from build123d import *

# Parameters (mm, degrees)
SKETCH1_W                       = 300
SKETCH1_H                       = 800
BOSS_EXTRUDE1_DEPTH             = 1
SKETCH2_W                       = 3
SKETCH2_H                       = 20
CUT_EXTRUDE1_DEPTH              = 10
EDGE_FLANGE1_STRIP_W            = 6
EDGE_FLANGE1_STRIP_H            = 1
EDGE_FLANGE1_STRIP_CUT_DEPTH    = 3
EDGE_FLANGE1_STRIP_2_W          = 6
EDGE_FLANGE1_STRIP_2_H          = 1
EDGE_FLANGE1_STRIP_CUT_2_DEPTH  = 3
EDGE_FLANGE1_STRIP_3_W          = 6
EDGE_FLANGE1_STRIP_3_H          = 1
EDGE_FLANGE1_STRIP_CUT_3_DEPTH  = 3
EDGE_FLANGE1_STRIP_4_W          = 6
EDGE_FLANGE1_STRIP_4_H          = 1
EDGE_FLANGE1_STRIP_CUT_4_DEPTH  = 3
EDGE_FLANGE1_STRIP_5_W          = 6
EDGE_FLANGE1_STRIP_5_H          = 1
EDGE_FLANGE1_STRIP_CUT_5_DEPTH  = 3
EDGE_FLANGE1_STRIP_6_W          = 6
EDGE_FLANGE1_STRIP_6_H          = 1
EDGE_FLANGE1_STRIP_CUT_6_DEPTH  = 3
EDGE_FLANGE1_STRIP_7_W          = 6
EDGE_FLANGE1_STRIP_7_H          = 1
EDGE_FLANGE1_STRIP_CUT_7_DEPTH  = 3
EDGE_FLANGE1_STRIP_8_W          = 6
EDGE_FLANGE1_STRIP_8_H          = 1
EDGE_FLANGE1_STRIP_CUT_8_DEPTH  = 3
EDGE_FLANGE1_STRIP_9_W          = 6
EDGE_FLANGE1_STRIP_9_H          = 1
EDGE_FLANGE1_STRIP_CUT_9_DEPTH  = 3
EDGE_FLANGE1_STRIP_10_W         = 6
EDGE_FLANGE1_STRIP_10_H         = 1
EDGE_FLANGE1_STRIP_CUT_10_DEPTH = 3
EDGE_FLANGE1_STRIP_11_W         = 6
EDGE_FLANGE1_STRIP_11_H         = 1
EDGE_FLANGE1_STRIP_CUT_11_DEPTH = 3
EDGE_FLANGE1_STRIP_12_W         = 6
EDGE_FLANGE1_STRIP_12_H         = 1
EDGE_FLANGE1_STRIP_CUT_12_DEPTH = 3
EDGE_FLANGE1_DEPTH              = 3
EDGE_FLANGE1_BEND_DEPTH         = 3
EDGE_FLANGE1_BEND_2_DEPTH       = 3
EDGE_FLANGE1_BEND_3_DEPTH       = 3
EDGE_FLANGE1_BEND_4_DEPTH       = 3
EDGE_FLANGE1_BEND_5_DEPTH       = 3
EDGE_FLANGE1_BEND_6_DEPTH       = 3
EDGE_FLANGE1_BEND_7_DEPTH       = 3
EDGE_FLANGE1_BEND_8_DEPTH       = 3
EDGE_FLANGE1_BEND_9_DEPTH       = 3
EDGE_FLANGE1_BEND_10_DEPTH      = 3
EDGE_FLANGE1_BEND_11_DEPTH      = 3


# Sheet-metal steps are written as plain solids
with BuildPart() as part:
    # Sketch1 → Boss-Extrude1 (new body)
    with BuildSketch(Plane.XY):
        Rectangle(SKETCH1_W, SKETCH1_H)
    extrude(amount=BOSS_EXTRUDE1_DEPTH)

    # Sketch2 → Cut-Extrude1 (cut)
    with BuildSketch(Plane.XY.offset(1)):
        with Locations((-140, 250)):
            Rectangle(SKETCH2_W, SKETCH2_H)
        with Locations((140, 250)):
            Rectangle(SKETCH2_W, SKETCH2_H)
        with Locations((140, 0)):
            Rectangle(SKETCH2_W, SKETCH2_H)
        with Locations((140, -250)):
            Rectangle(SKETCH2_W, SKETCH2_H)
        with Locations((-140, 0)):
            Rectangle(SKETCH2_W, SKETCH2_H)
        with Locations((-140, -250)):
            Rectangle(SKETCH2_W, SKETCH2_H)
    extrude(amount=-CUT_EXTRUDE1_DEPTH, mode=Mode.SUBTRACT)

    # Edge-Flange1 strip (across the edge) → Edge-Flange1 strip cut (cut)
    with BuildSketch(Plane(origin=(-138.5, 260, 0), x_dir=(0, 1, 0), z_dir=(-1, 0, 0))):
        with Locations((-2, -0.5)):
            Rectangle(EDGE_FLANGE1_STRIP_W, EDGE_FLANGE1_STRIP_H)
    extrude(amount=EDGE_FLANGE1_STRIP_CUT_DEPTH, mode=Mode.SUBTRACT)

    # Edge-Flange1 strip 2 (across the edge) → Edge-Flange1 strip cut 2 (cut)
    with BuildSketch(Plane(origin=(-141.5, 240, 0), x_dir=(0, -1, 0), z_dir=(1, 0, 0))):
        with Locations((-2, -0.5)):
            Rectangle(EDGE_FLANGE1_STRIP_2_W, EDGE_FLANGE1_STRIP_2_H)
    extrude(amount=EDGE_FLANGE1_STRIP_CUT_2_DEPTH, mode=Mode.SUBTRACT)

    # Edge-Flange1 strip 3 (across the edge) → Edge-Flange1 strip cut 3 (cut)
    with BuildSketch(Plane(origin=(141.5, 260, 0), x_dir=(0, 1, 0), z_dir=(-1, 0, 0))):
        with Locations((-2, -0.5)):
            Rectangle(EDGE_FLANGE1_STRIP_3_W, EDGE_FLANGE1_STRIP_3_H)
    extrude(amount=EDGE_FLANGE1_STRIP_CUT_3_DEPTH, mode=Mode.SUBTRACT)

    # Edge-Flange1 strip 4 (across the edge) → Edge-Flange1 strip cut 4 (cut)
    with BuildSketch(Plane(origin=(138.5, 240, 0), x_dir=(0, -1, 0), z_dir=(1, 0, 0))):
        with Locations((-2, -0.5)):
            Rectangle(EDGE_FLANGE1_STRIP_4_W, EDGE_FLANGE1_STRIP_4_H)
    extrude(amount=EDGE_FLANGE1_STRIP_CUT_4_DEPTH, mode=Mode.SUBTRACT)

    # Edge-Flange1 strip 5 (across the edge) → Edge-Flange1 strip cut 5 (cut)
    with BuildSketch(Plane(origin=(-141.5, -10, 0), x_dir=(0, -1, 0), z_dir=(1, 0, 0))):
        with Locations((-2, -0.5)):
            Rectangle(EDGE_FLANGE1_STRIP_5_W, EDGE_FLANGE1_STRIP_5_H)
    extrude(amount=EDGE_FLANGE1_STRIP_CUT_5_DEPTH, mode=Mode.SUBTRACT)

    # Edge-Flange1 strip 6 (across the edge) → Edge-Flange1 strip cut 6 (cut)
    with BuildSketch(Plane(origin=(138.5, -10, 0), x_dir=(0, -1, 0), z_dir=(1, 0, 0))):
        with Locations((-2, -0.5)):
            Rectangle(EDGE_FLANGE1_STRIP_6_W, EDGE_FLANGE1_STRIP_6_H)
    extrude(amount=EDGE_FLANGE1_STRIP_CUT_6_DEPTH, mode=Mode.SUBTRACT)

    # Edge-Flange1 strip 7 (across the edge) → Edge-Flange1 strip cut 7 (cut)
    with BuildSketch(Plane(origin=(-141.5, -260, 0), x_dir=(0, -1, 0), z_dir=(1, 0, 0))):
        with Locations((-2, -0.5)):
            Rectangle(EDGE_FLANGE1_STRIP_7_W, EDGE_FLANGE1_STRIP_7_H)
    extrude(amount=EDGE_FLANGE1_STRIP_CUT_7_DEPTH, mode=Mode.SUBTRACT)

    # Edge-Flange1 strip 8 (across the edge) → Edge-Flange1 strip cut 8 (cut)
    with BuildSketch(Plane(origin=(138.5, -260, 0), x_dir=(0, -1, 0), z_dir=(1, 0, 0))):
        with Locations((-2, -0.5)):
            Rectangle(EDGE_FLANGE1_STRIP_8_W, EDGE_FLANGE1_STRIP_8_H)
    extrude(amount=EDGE_FLANGE1_STRIP_CUT_8_DEPTH, mode=Mode.SUBTRACT)

    # Edge-Flange1 strip 9 (across the edge) → Edge-Flange1 strip cut 9 (cut)
    with BuildSketch(Plane(origin=(141.5, -240, 0), x_dir=(0, 1, 0), z_dir=(-1, 0, 0))):
        with Locations((-2, -0.5)):
            Rectangle(EDGE_FLANGE1_STRIP_9_W, EDGE_FLANGE1_STRIP_9_H)
    extrude(amount=EDGE_FLANGE1_STRIP_CUT_9_DEPTH, mode=Mode.SUBTRACT)

    # Edge-Flange1 strip 10 (across the edge) → Edge-Flange1 strip cut 10 (cut)
    with BuildSketch(Plane(origin=(141.5, 10, 0), x_dir=(0, 1, 0), z_dir=(-1, 0, 0))):
        with Locations((-2, -0.5)):
            Rectangle(EDGE_FLANGE1_STRIP_10_W, EDGE_FLANGE1_STRIP_10_H)
    extrude(amount=EDGE_FLANGE1_STRIP_CUT_10_DEPTH, mode=Mode.SUBTRACT)

    # Edge-Flange1 strip 11 (across the edge) → Edge-Flange1 strip cut 11 (cut)
    with BuildSketch(Plane(origin=(-138.5, 10, 0), x_dir=(0, 1, 0), z_dir=(-1, 0, 0))):
        with Locations((-2, -0.5)):
            Rectangle(EDGE_FLANGE1_STRIP_11_W, EDGE_FLANGE1_STRIP_11_H)
    extrude(amount=EDGE_FLANGE1_STRIP_CUT_11_DEPTH, mode=Mode.SUBTRACT)

    # Edge-Flange1 strip 12 (across the edge) → Edge-Flange1 strip cut 12 (cut)
    with BuildSketch(Plane(origin=(-138.5, -240, 0), x_dir=(0, 1, 0), z_dir=(-1, 0, 0))):
        with Locations((-2, -0.5)):
            Rectangle(EDGE_FLANGE1_STRIP_12_W, EDGE_FLANGE1_STRIP_12_H)
    extrude(amount=EDGE_FLANGE1_STRIP_CUT_12_DEPTH, mode=Mode.SUBTRACT)

    # Edge-Flange1 section (across the edge) → Edge-Flange1 (add)
    with BuildSketch(Plane(origin=(-138.5, 260, 0), x_dir=(0, 1, 0), z_dir=(-1, 0, 0))):
        with BuildLine():
            Line((-1, 1), (-1, 10))
            Line((-1, 10), (0, 10))
            Line((0, 10), (0, 1))
            ThreePointArc((0, 1), (0.292893219, 0.292893219), (1, 0))
            Line((1, 0), (1, -1))
            ThreePointArc((1, -1), (-0.414213562, -0.414213562), (-1, 1))
        make_face()
    extrude(amount=EDGE_FLANGE1_DEPTH)

    # Edge-Flange1 section 2 (across the edge) → Edge-Flange1 bend (add)
    with BuildSketch(Plane(origin=(-141.5, 240, 0), x_dir=(0, -1, 0), z_dir=(1, 0, 0))):
        with BuildLine():
            Line((-1, 1), (-1, 10))
            Line((-1, 10), (0, 10))
            Line((0, 10), (0, 1))
            ThreePointArc((0, 1), (0.292893219, 0.292893219), (1, 0))
            Line((1, 0), (1, -1))
            ThreePointArc((1, -1), (-0.414213562, -0.414213562), (-1, 1))
        make_face()
    extrude(amount=EDGE_FLANGE1_BEND_DEPTH)

    # Edge-Flange1 section 3 (across the edge) → Edge-Flange1 bend 2 (add)
    with BuildSketch(Plane(origin=(141.5, 260, 0), x_dir=(0, 1, 0), z_dir=(-1, 0, 0))):
        with BuildLine():
            Line((-1, 1), (-1, 10))
            Line((-1, 10), (0, 10))
            Line((0, 10), (0, 1))
            ThreePointArc((0, 1), (0.292893219, 0.292893219), (1, 0))
            Line((1, 0), (1, -1))
            ThreePointArc((1, -1), (-0.414213562, -0.414213562), (-1, 1))
        make_face()
    extrude(amount=EDGE_FLANGE1_BEND_2_DEPTH)

    # Edge-Flange1 section 4 (across the edge) → Edge-Flange1 bend 3 (add)
    with BuildSketch(Plane(origin=(138.5, 240, 0), x_dir=(0, -1, 0), z_dir=(1, 0, 0))):
        with BuildLine():
            Line((-1, 1), (-1, 10))
            Line((-1, 10), (0, 10))
            Line((0, 10), (0, 1))
            ThreePointArc((0, 1), (0.292893219, 0.292893219), (1, 0))
            Line((1, 0), (1, -1))
            ThreePointArc((1, -1), (-0.414213562, -0.414213562), (-1, 1))
        make_face()
    extrude(amount=EDGE_FLANGE1_BEND_3_DEPTH)

    # Edge-Flange1 section 5 (across the edge) → Edge-Flange1 bend 4 (add)
    with BuildSketch(Plane(origin=(-141.5, -10, 0), x_dir=(0, -1, 0), z_dir=(1, 0, 0))):
        with BuildLine():
            Line((-1, 1), (-1, 10))
            Line((-1, 10), (0, 10))
            Line((0, 10), (0, 1))
            ThreePointArc((0, 1), (0.292893219, 0.292893219), (1, 0))
            Line((1, 0), (1, -1))
            ThreePointArc((1, -1), (-0.414213562, -0.414213562), (-1, 1))
        make_face()
    extrude(amount=EDGE_FLANGE1_BEND_4_DEPTH)

    # Edge-Flange1 section 6 (across the edge) → Edge-Flange1 bend 5 (add)
    with BuildSketch(Plane(origin=(138.5, -10, 0), x_dir=(0, -1, 0), z_dir=(1, 0, 0))):
        with BuildLine():
            Line((-1, 1), (-1, 10))
            Line((-1, 10), (0, 10))
            Line((0, 10), (0, 1))
            ThreePointArc((0, 1), (0.292893219, 0.292893219), (1, 0))
            Line((1, 0), (1, -1))
            ThreePointArc((1, -1), (-0.414213562, -0.414213562), (-1, 1))
        make_face()
    extrude(amount=EDGE_FLANGE1_BEND_5_DEPTH)

    # Edge-Flange1 section 7 (across the edge) → Edge-Flange1 bend 6 (add)
    with BuildSketch(Plane(origin=(-141.5, -260, 0), x_dir=(0, -1, 0), z_dir=(1, 0, 0))):
        with BuildLine():
            Line((-1, 1), (-1, 10))
            Line((-1, 10), (0, 10))
            Line((0, 10), (0, 1))
            ThreePointArc((0, 1), (0.292893219, 0.292893219), (1, 0))
            Line((1, 0), (1, -1))
            ThreePointArc((1, -1), (-0.414213562, -0.414213562), (-1, 1))
        make_face()
    extrude(amount=EDGE_FLANGE1_BEND_6_DEPTH)

    # Edge-Flange1 section 8 (across the edge) → Edge-Flange1 bend 7 (add)
    with BuildSketch(Plane(origin=(138.5, -260, 0), x_dir=(0, -1, 0), z_dir=(1, 0, 0))):
        with BuildLine():
            Line((-1, 1), (-1, 10))
            Line((-1, 10), (0, 10))
            Line((0, 10), (0, 1))
            ThreePointArc((0, 1), (0.292893219, 0.292893219), (1, 0))
            Line((1, 0), (1, -1))
            ThreePointArc((1, -1), (-0.414213562, -0.414213562), (-1, 1))
        make_face()
    extrude(amount=EDGE_FLANGE1_BEND_7_DEPTH)

    # Edge-Flange1 section 9 (across the edge) → Edge-Flange1 bend 8 (add)
    with BuildSketch(Plane(origin=(141.5, -240, 0), x_dir=(0, 1, 0), z_dir=(-1, 0, 0))):
        with BuildLine():
            Line((-1, 1), (-1, 10))
            Line((-1, 10), (0, 10))
            Line((0, 10), (0, 1))
            ThreePointArc((0, 1), (0.292893219, 0.292893219), (1, 0))
            Line((1, 0), (1, -1))
            ThreePointArc((1, -1), (-0.414213562, -0.414213562), (-1, 1))
        make_face()
    extrude(amount=EDGE_FLANGE1_BEND_8_DEPTH)

    # Edge-Flange1 section 10 (across the edge) → Edge-Flange1 bend 9 (add)
    with BuildSketch(Plane(origin=(141.5, 10, 0), x_dir=(0, 1, 0), z_dir=(-1, 0, 0))):
        with BuildLine():
            Line((-1, 1), (-1, 10))
            Line((-1, 10), (0, 10))
            Line((0, 10), (0, 1))
            ThreePointArc((0, 1), (0.292893219, 0.292893219), (1, 0))
            Line((1, 0), (1, -1))
            ThreePointArc((1, -1), (-0.414213562, -0.414213562), (-1, 1))
        make_face()
    extrude(amount=EDGE_FLANGE1_BEND_9_DEPTH)

    # Edge-Flange1 section 11 (across the edge) → Edge-Flange1 bend 10 (add)
    with BuildSketch(Plane(origin=(-138.5, 10, 0), x_dir=(0, 1, 0), z_dir=(-1, 0, 0))):
        with BuildLine():
            Line((-1, 1), (-1, 10))
            Line((-1, 10), (0, 10))
            Line((0, 10), (0, 1))
            ThreePointArc((0, 1), (0.292893219, 0.292893219), (1, 0))
            Line((1, 0), (1, -1))
            ThreePointArc((1, -1), (-0.414213562, -0.414213562), (-1, 1))
        make_face()
    extrude(amount=EDGE_FLANGE1_BEND_10_DEPTH)

    # Edge-Flange1 section 12 (across the edge) → Edge-Flange1 bend 11 (add)
    with BuildSketch(Plane(origin=(-138.5, -240, 0), x_dir=(0, 1, 0), z_dir=(-1, 0, 0))):
        with BuildLine():
            Line((-1, 1), (-1, 10))
            Line((-1, 10), (0, 10))
            Line((0, 10), (0, 1))
            ThreePointArc((0, 1), (0.292893219, 0.292893219), (1, 0))
            Line((1, 0), (1, -1))
            ThreePointArc((1, -1), (-0.414213562, -0.414213562), (-1, 1))
        make_face()
    extrude(amount=EDGE_FLANGE1_BEND_11_DEPTH)


solid = part.part
For this review, take the finished solid that the model builds, in its own axes (mm). Round coordinates to 2 decimals unless told otherwise and drop trailing zeros. Loops run counter-clockwise (first coordinate to the right, second up) from the corner with the lowest first, then second, coordinate; pieces in that order, holes last. Notation, with made-up numbers: (25.25, 26) - (61.25, 26) arc R25 cw to (61.25, 41) - close; hole circle Ø7 at (54.25, 15). An arc over 180 degrees is marked (long way). One line per item, written item: value. Start each with the question number.
Item 1: Take a section at C-C (x = -28). Give the boundary of the cut face in (y, z), plus the area to 3 significant figures.
Item 2: Take a section at D-D (y = -336.5). Give the boundary of the cut face in (x, z), plus the area to 3 significant figures.
Item 3: Clearance check with flat-ended pins moving along their axes: pin 1 Ø1.5 at (x, z) = (-140, -5.5) entering from -Y; pin 2 Ø4 at (x, z) = (10, -1.5) entering from +Y; pin 3 Ø1.6 at (y, z) = (260.5, -3.5) entering from -X; pin 4 Ø0.6 at (y, z) = (-260.5, -3) entering from +X. State where each tip first meets the part, or that it passes through.
Item 4: For L1, parallel to Z at x = -11, y = -88.5, list the stretches that pass through material, from the lowest coordinate up.
Item 5: Take a section at B-B (z = -8.25). State how many separate pieces and enclosed holes the cut face has, plus the area to 3 significant figures.
Item 6: Take a section at A-A (y = -248). Give the boundary of the cut face in (x, z), plus the area to 3 significant figures.
Answer below:
1. outline: (-400, 0) - (400, 0) - (400, 1) - (-400, 1) - close
1. area: 800 mm2
2. outline: (-150, 0) - (150, 0) - (150, 1) - (-150, 1) - close
2. area: 300 mm2
3. pin 1: stops at y = -260
3. pin 2: stops at y = 400
3. pin 3: stops at x = -141.5
3. pin 4: passes through
4. L1: z = 0 to 1
5. separate pieces: 12
5. enclosed holes: 0
5. area: 36.0 mm2
6. outline: (-150, 0) - (-141.5, 0) - (-141.5, 1) - (-150, 1) - close; (-138.5, 0) - (138.5, 0) - (138.5, 1) - (-138.5, 1) - close; (141.5, 0) - (150, 0) - (150, 1) - (141.5, 1) - close
6. area: 294 mm2
